Check sheet for the modelled part. Datum: model origin and axes. Units: mm. Give positions to 0.01 mm unless a question says otherwise; leave off trailing zeros. Loops run counter-clockwise (first coordinate to the right, second up) from the corner with the lowest first, then second, coordinate; pieces in that order, holes last. Notation, with made-up numbers: (24, -8.75) -> (35, -8.75) arc R17 ccw to (35, -2.75) -> close; hole circle Ø10 at (74.5, -39). An arc over 180 degrees is marked (long way). Answer as CSV lines item,"result". Start each with the question number.
(1) Section check A-A on x = 32.5. Enter the section's corners in (y, z), plus the area to 3 significant figures.
(2) Material ranges on line 1 (X direction, y = 0, z = 4.75); line 2 (X direction, y = 0, z = 3.2); line 3 (Y direction, x = -22.5, z = 2.6), recorded low to high. Write a range as from..to.
(3) Gauge pin test, flat ends, axial feed: pin 1 Ø2 at (x, y) = (32.5, 0) entering from +Z; pin 2 Ø2.5 at (x, y) = (22.5, 0) entering from +Z; pin 3 Ø3.5 at (x, y) = (32.5, 0) entering from +Z. Record the tip position at first contact, or that the pin passes through.
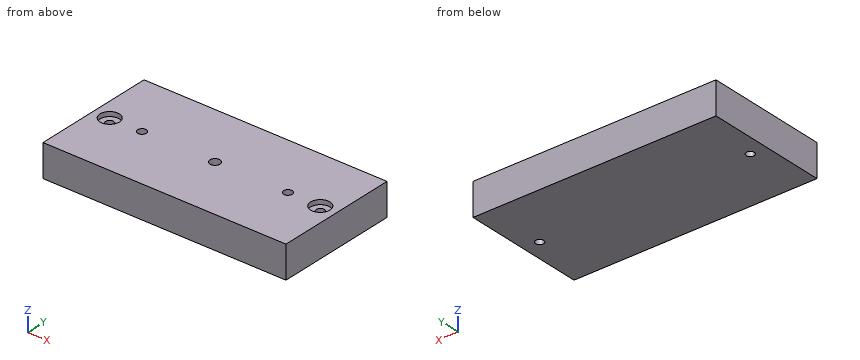
Autodesk Inventor part; units mm, degrees
ref_plane "YZ Plane" through (0, 0, 0) normal (1, 0, 0) x (0, 1, 0)
ref_plane "XZ Plane" through (0, 0, 0) normal (0, 1, 0) x (-1, 0, 0)
ref_plane "XY Plane" through (0, 0, 0) normal (0, 0, 1) x (1, 0, 0)
sketch "Sketch1" plane through (0, 0, 0) normal (0, 0, 1) x (1, 0, 0)
  line L0 (-37.5, 19) -> (37.5, 19)
  line L1 (37.5, 19) -> (37.5, -19)
  line L2 (37.5, -19) -> (-37.5, -19)
  line L3 (-37.5, -19) -> (-37.5, 19)
  line L4 (-37.5, 19) -> (37.5, -19) construction
  line L5 (37.5, 19) -> (-37.5, -19) construction
  point P0 (0, 0)
  dimension "d2" = 38
  dimension "d3" = 75
extrude "Extrusion1" add sketch "Sketch1" along normal mid plane 10
sketch "Sketch3" plane through (0, 0, 5) normal (0, 0, 1) x (1, 0, 0)
  point P0 (0, 0)
  point P1 (0, 0)
hole "Hole2" at (0, 0, 5) direction (0, 0, -1) diameter 3.175 depth 5 tip angle 118
sketch "Sketch4" plane through (0, 0, 5) normal (0, 0, 1) x (1, 0, 0)
  line L0 (-37.5, 19) -> (-37.5, -19)
  circle A0 centre (0, 0) radius 1.5875
  line L1 (-37.5, -19) -> (37.5, -19)
  line L2 (37.5, -19) -> (37.5, 19)
  line L3 (37.5, 19) -> (-37.5, 19)
  line L4 (-37.5, 19) -> (-37.5, -19)
  point P0 (-32.5, 0)
  point P1 (32.5, 0)
  dimension "d76" = 5
  dimension "d79" = 65
hole "Hole3" at (-32.5, 0, 5) at (32.5, 0, 5) direction (0, 0, -1) diameter 2.459 end through all counterbore diameter 6 counterbore depth 1.4
sketch "Sketch5" plane through (0, 0, 5) normal (0, 0, 1) x (1, 0, 0)
  point P0 (0, 0)
  point P1 (-22.5, 0)
  point P2 (22.5, 0)
  dimension "d95" = 22.5
  dimension "d96" = 22.5
hole "Hole4" at (-22.5, 0, 5) at (22.5, 0, 5) direction (0, 0, -1) diameter 2.7 depth 3 tip angle 118
properties part number "baseblock"
Working result:
1,outline,"(-19, -5) -> (-1.23, -5) -> (-1.23, 3.6) -> (-3, 3.6) -> (-3, 5) -> (-19, 5) -> close; (1.23, -5) -> (19, -5) -> (19, 5) -> (3, 5) -> (3, 3.6) -> (1.23, 3.6) -> close"
1,area,"350 mm^2"
2,line 1,"x = -37.5..-35.5, -29.5..-23.85, -21.15..-1.59, 1.59..21.15, 23.85..29.5, 35.5..37.5"
2,line 2,"x = -37.5..-33.73, -31.27..-23.85, -21.15..-1.59, 1.59..21.15, 23.85..31.27, 33.73..37.5"
2,line 3,"y = -19..-1.35, 1.35..19"
3,pin 1,"passes through"
3,pin 2,"stops at z = 1.94"
3,pin 3,"stops at z = 3.6"
